from build123d import *

# Parameters (mm, degrees)
SKETCH1_R           = 36.40455
BOSS_EXTRUDE1_DEPTH = 197.64375
SKETCH2_R           = 33.274
BOSS_EXTRUDE2_DEPTH = 6.7818
SKETCH3_R           = 27.2288
BOSS_EXTRUDE3_DEPTH = 13.97
SHELL1_T            = -3.048
FILLET1_R           = 3.81
FILLET2_R           = 2.54
FILLET3_R           = 1
FILLET4_R           = 1.000000032


with BuildPart() as part:
    # Sketch1 → Boss-Extrude1 (new body)
    with BuildSketch(Plane.XY):
        with Locations(Location((0, 0, 0), (0, 0, 180))):
            Circle(SKETCH1_R)
    extrude(amount=BOSS_EXTRUDE1_DEPTH)

    # Sketch2 → Boss-Extrude2 (add)
    with BuildSketch(Plane.XY.offset(197.64375)):
        with Locations(Location((0, 0, 0), (0, 0, 180))):
            Circle(SKETCH2_R)
    extrude(amount=BOSS_EXTRUDE2_DEPTH)

    # Sketch3 → Boss-Extrude3 (add)
    with BuildSketch(Plane.XY.offset(204.42555)):
        Circle(SKETCH3_R)
    extrude(amount=BOSS_EXTRUDE3_DEPTH)

    # Shell1
    shell1_openings = [part.faces().sort_by_distance(p)[0] for p in [
        (0, 0, 218.39555),
    ]]
    offset(amount=SHELL1_T, openings=shell1_openings, kind=Kind.INTERSECTION)

    # Fillet1
    # the kernel refuses this fillet: 3.81 mm, written as the material it takes off along each edge
    with BuildSketch(Plane(origin=(0, 0, 197.64375), x_dir=(-1, 0, 0), z_dir=(0, 1, 0))) as fillet1_piece_1:
        with BuildLine():
            CenterArc((32.59455, -3.748926206), FILLET1_R, 0, 79.727303784)
            Line((33.274, 0), (33.287589, 0.074978524))
            ThreePointArc((33.287589, 0.074978524), (34.839275, 0.0762), (36.40455, 0.0762))
            Line((36.40455, 0.0762), (36.48075, 0))
            Line((36.48075, 0), (36.48075, -3.748926206))
            Line((36.48075, -3.748926206), (36.40455, -3.748926206))
        make_face()
    revolve(axis=Axis((0, 0, 197.64375), (0, 0, 1)), mode=Mode.SUBTRACT)

    # Fillet2
    fillet2_edges = [part.edges().sort_by_distance(p)[0] for p in [
        (33.274, 0, 204.42555),
    ]]
    fillet(fillet2_edges, radius=FILLET2_R)

    # Fillet3
    fillet3_edges = [part.edges().sort_by_distance(p)[0] for p in [
        (-27.2288, 0, 204.42555),
    ]]
    fillet(fillet3_edges, radius=FILLET3_R)

    # Fillet4
    fillet4_edges = [part.edges().sort_by_distance(p)[0] for p in [
        (-27.2288, 0, 218.39555),
        (-24.1808, 0, 218.39555),
    ]]
    fillet(fillet4_edges, radius=FILLET4_R)


solid = part.part
Work out the finished part from the listing and answer in its coordinate system (mm). A direction names the side the tool comes from. Round coordinates to 2 decimals unless told otherwise and drop trailing zeros. Write each loop counter-clockwise with the first axis right and the second up, starting at its lowest first coordinate (ties: lowest second). Pieces come first, ordered by that corner, then holes. Notation, with made-up numbers: (2.5, 87.5) -> (42.5, 87.5) arc R6 cw to (42.5, 92.5) -> close; hole circle Ø5 at (19.25, 20.25). An arc over 180 degrees is marked (long way). Answer as CSV lines item,"result". Start each with the question number.
(1) The mould has two halves that part along Y. Classify faces 4 (the cylindrical face through (-34.723, -10.935, 95.59)), 5 (the cylindrical face through (-19.2, -14.7, 209.3)), 6 (the flat face through (30, -5, 194.596)), 7 (the flat face through (1, -1, 0)): +Y half, -Y half, draft (parallel to the pull), parting line (faces both ways), or undercut.
(2) Find the intervals of material crossed by probe 1 along Y at (x, z) = (0, 151); probe 2 along Y at (x, z) = (0, 212.5); probe 3 along Z at (x, y) = (23.5, 9), in increasing order.
(3) Each of these flat-tipped pins is pushed along its axis until it touches: pin 1 (5 mm diameter, centred on x = -18, z = 82.5, fed in from +Y); pin 2 (1.5 mm diameter, centred on y = -15.5, z = 164.5, fed in from +X); pin 3 (4 mm diameter, centred on x = -11.5, z = 82, fed in from -Y). Where does it stop, or does it pass through?
(4) A tool of negligible diameter and unlimited length cuts with its end or side. For faces 1 (the cylindrical face through (4.33, -32.99, 199.73)), 2 (the flat face through (-9.8, 23.4, 218.396)), 3 (the flat face through (0, 0, 3.048)), from which of +Z, -Z, +X, -X, +Y, -Y can it reach the whole face along a straight path? Write none if from no direction.
(5) The part is cut by section C-C, the plane z = 129. Give the vertices of the cut face in (x, y).
Output values:
1,face 4,"parting line"
1,face 5,"undercut"
1,face 6,"undercut"
1,face 7,"draft"
2,probe 1,"y = -36.4 to -33.36, 33.36 to 36.4"
2,probe 2,"y = -27.23 to -24.18, 24.18 to 27.23"
2,probe 3,"z = 0 to 3.05, 201.38 to 218.4"
3,pin 1,"stops at y = 32.94"
3,pin 2,"stops at x = 33.28"
3,pin 3,"stops at y = -35.14"
4,face 1,"+Z"
4,face 2,"+Z, +X, -X, +Y, -Y"
4,face 3,"none"
5,outline,"circle Ø72.81 at (0, 0); hole circle Ø66.71 at (0, 0)"
